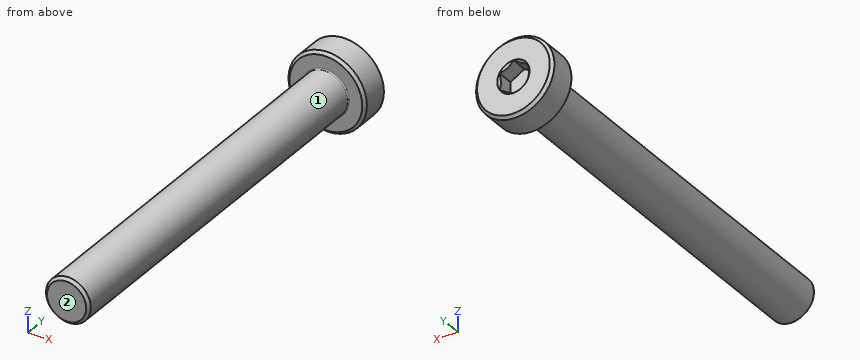
Autodesk Inventor part; units mm, degrees
ref_plane "YZ Plane" through (0, 0, 0) normal (1, 0, 0) x (0, 1, 0)
ref_plane "XZ Plane" through (0, 0, 0) normal (0, 1, 0) x (-1, 0, 0)
ref_plane "XY Plane" through (0, 0, 0) normal (0, 0, 1) x (1, 0, 0)
sketch "Sketch1" plane through (0, 0, 0) normal (0, 0, 1) x (1, 0, 0)
  line L0 (0, 18.9) -> (0, -18.9)
  line L1 (0, -18.9) -> (1.75, -18.9)
  line L2 (1.75, -18.9) -> (2, -18.65)
  line L3 (2, -18.65) -> (2, 16)
  line L4 (2.1, 16.1) -> (3.25, 16.1)
  line L5 (3.5, 16.35) -> (3.5, 18.65)
  line L6 (3.25, 18.9) -> (0, 18.9)
  arc A0 (2.1, 16.1) -> (2, 16) centre (2.1, 16) ccw
  line L7 (3.25, 18.9) -> (3.5, 18.65)
  line L8 (3.25, 16.1) -> (3.5, 16.35)
  point P0 (0, 0)
  point P1 (3.5, 16.1)
  point P2 (3.5, 18.9)
  point P3 (0, 0)
  dimension "d0" = 7
  dimension "d1" = 2.8
  dimension "d3" = 4
  dimension "d4" = 4.2
  dimension "d5" = 135
  dimension "d6" = 0.25
  dimension "d7" = 35
  dimension "d9" = 0.25
revolve "Revolution1" add sketch "Sketch1" angle 360 about axis through (0, 18.9, 0) along (0, -1, 0)
sketch "Sketch2" plane through (0, 18.9, 0) normal (0, 1, 0) x (1, 0, 0)
  line L0 (0, -1.4434) -> (-1.25, -0.7217)
  line L1 (-1.25, -0.7217) -> (-1.25, 0.7217)
  line L2 (-1.25, 0.7217) -> (0, 1.4434)
  line L3 (0, 1.4434) -> (1.25, 0.7217)
  line L4 (1.25, 0.7217) -> (1.25, -0.7217)
  line L5 (1.25, -0.7217) -> (0, -1.4434)
  point P0 (0, 0)
  point P1 (0, 0)
  dimension "d11" = 2.5
extrude "Extrusion1" cut sketch "Sketch2" against normal blind 1.5
thread "Thread1"
sketch "Sketch3" plane through (0, 0, 0) normal (1, 0, 0) x (0, 1, 0)
  line L0 (18.9, 1.4434) -> (17.9, 0.4434)
  line L1 (17.9, 0.4434) -> (18.9, 0.4434)
  line L2 (18.9, 0.4434) -> (18.9, 1.4434)
  line L3 (-1.4, 0) -> (8.4, 0)
  point P0 (0, 0)
  dimension "d18" = 1
revolve "Revolution2" cut sketch "Sketch3" angle 360 about axis through (0, -10, 0) along (0, 1, 0)
properties part number "Bolt_M4x0.7_35mm_LSH" material "Stainless Steel"
Geometry: final body of the model. Coordinates: model frame, mm. Face numbers are marked on the shaded views. A direction names the side the tool comes from. Give positions to 0.01 mm unless a question says otherwise; leave off trailing zeros. Loops run counter-clockwise (first coordinate to the right, second up) from the corner with the lowest first, then second, coordinate; pieces in that order, holes last. Notation, with made-up numbers: (40.25, 51) -> (96.25, 51) arc R21 ccw to (96.25, 55) -> close; hole circle Ø5 at (72.5, 67.5). An arc over 180 degrees is marked (long way). Put each result on its own line as item: value.
1. Ray query, line 1 along Y through (x, z) = (0, -2.75); line 2 along Y through (x, z) = (0, 0.25); line 3 along X through (y, z) = (-2, 1.5). Return the intervals inside material, ascending. Write a range as [from, to].
Taken from the geometry:
line 1: y = [16.1, 18.9]
line 2: y = [-18.9, 17.4]
line 3: x = [-1.32, 1.32]
2. Pin query (flat end, axial travel): P1, Ø3, axis at y = 12.5, z = -0.5, coming from the -X side; P2, Ø0.8, axis at x = 0, z = 0.5, coming from the +Y side; P3, Ø1, axis at y = 5.5, z = -2, coming from the -X side. Return the tip coordinate at first contact, or that it passes through.
Taken from the geometry:
P1: stops at x = -2
P2: stops at y = 17.4
P3: stops at x = -1.32
3. Cut plane A-A (z = 0). Return the cut outline in (x, y), plus the area to 3 significant figures.
Taken from the geometry:
outline: (-3.5, 16.35) -> (-3.25, 16.1) -> (-2.1, 16.1) arc R0.1 cw to (-2, 16) -> (-2, -18.65) -> (-1.75, -18.9) -> (1.75, -18.9) -> (2, -18.65) -> (2, 16) arc R0.1 cw to (2.1, 16.1) -> (3.25, 16.1) -> (3.5, 16.35) -> (3.5, 18.65) -> (3.25, 18.9) -> (1.44, 18.9) -> (1.25, 18.71) -> (1.25, 17.4) -> (-1.25, 17.4) -> (-1.25, 18.71) -> (-1.44, 18.9) -> (-3.25, 18.9) -> (-3.5, 18.65) -> close
area: 156 mm2
4. Set-up query: the marked faces 1 and 2. Return all of +Z, -Z, +X, -X, +Y, -Y with unobstructed straight access to the full face (end or side cutting, diameter ignored); none if empty.
Taken from the geometry:
face 1: -Y
face 2: +Z, -Z, +X, -X, -Y
5. Cut plane B-B (y = 0.5). Return the cut outline in (x, z).
Taken from the geometry:
outline: circle Ø4 at (0, 0)
